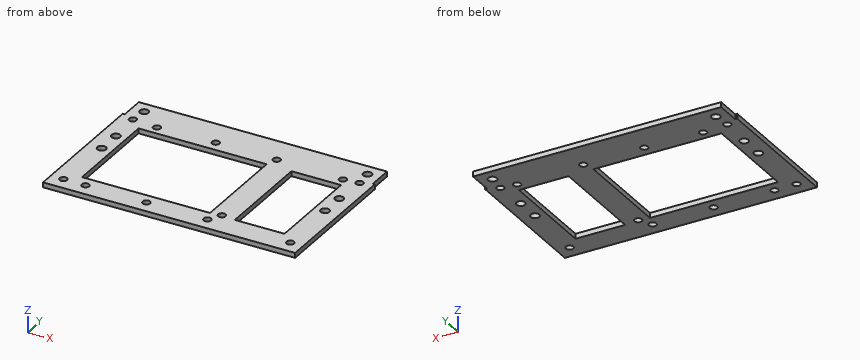
from build123d import *

# Parameters (mm, degrees)
F0_W      = 101.6
F0_H      = 53.34
F1_DEPTH  = 2
F3_D      = 3
F4_W      = 101.6
F4_H      = 3
F4_W_2    = 100
F4_H_2    = 10
F5_DEPTH  = 2
F7_D      = 3.5
F9_D      = 3
F10_W     = 51.6
F10_H     = 40
F10_W_2   = 20
F11_DEPTH = 2.001


with BuildPart() as f1:
    # F0 (on Top) → F1 (new body)
    with BuildSketch(Plane.XY):
        Rectangle(F0_W, F0_H)
    extrude(amount=F1_DEPTH)

    # F3 (through all)
    with Locations(Plane.XY.offset(2)):
        with Locations((-35.56, 24.13), (39.37, 24.13), (45.72, -24.13), (15.24, -19.05), (-36.83, -24.13)):
            Hole(F3_D / 2)

    # F4 (on face) → F5 (join, through all)
    with BuildSketch(Plane.XY.offset(2)):
        with Locations((0, -28.17)):
            Rectangle(F4_W, F4_H)
        with Locations((0, 31.67)):
            Rectangle(F4_W_2, F4_H_2)
    extrude(amount=-F5_DEPTH)

    # F7 (through all)
    with Locations(Plane.XY.offset(2)):
        with Locations((-45, 31.67), (45, 31.67), (-45, 11.67), (-45, 1.67), (45, 11.67), (45, 1.67)):
            Hole(F7_D / 2)

    # F9 (through all)
    with Locations(Plane.XY.offset(2)):
        with Locations((-45.72, -24.13), (-45.72, 24.87), (-12.28, 24.87), (12.28, 24.87), (12.28, -24.13), (-12.28, -24.13), (45.72, 24.87)):
            Hole(F9_D / 2)

    # F10 (on face) → F11 (cut, through all)
    with BuildSketch(Plane(origin=(0, 0, 0), x_dir=(1, 0, 0), z_dir=(0, 0, -1))):
        with Locations((-15, -0.33)):
            Rectangle(F10_W, F10_H)
        with Locations((30.8, -0.33)):
            Rectangle(F10_W_2, F10_H)
    extrude(amount=-F11_DEPTH, mode=Mode.SUBTRACT)


solid = f1.part
Read the model definition and answer for the solid it produces. Units are mm, in the model's axes. Coordinates: 2 decimals unless noted, no trailing zeros. Write each loop counter-clockwise with the first axis right and the second up, starting at its lowest first coordinate (ties: lowest second). Pieces come first, ordered by that corner, then holes. Notation, with made-up numbers: (14.5, 9) - (69.5, 9) arc R18 ccw to (69.5, 13) - close; hole circle Ø10 at (78.5, 18.25). An arc over 180 degrees is marked (long way). One line per question, with ' | ' between items.
Q1. Find section D-D, the plane y = 1.67. Write down the section's boundary in (x, z), plus the area to 3 significant figures.
Result set:
outline: (-50.8, 0) - (-46.75, 0) - (-46.75, 2) - (-50.8, 2) - close; (-43.25, 0) - (-40.8, 0) - (-40.8, 2) - (-43.25, 2) - close; (10.8, 0) - (20.8, 0) - (20.8, 2) - (10.8, 2) - close; (40.8, 0) - (43.25, 0) - (43.25, 2) - (40.8, 2) - close; (46.75, 0) - (50.8, 0) - (50.8, 2) - (46.75, 2) - close | area: 46.0 mm^2
Q2. Each of these flat-tipped pins is pushed along its axis until it touches: P1, Ø6, axis at x = -37, y = -0.5, coming from the -Z side; P2, Ø0.6, axis at x = -50.5, z = 0.5, coming from the +Y side. Where does it stop, or does it pass through?
Result set:
P1: through | P2: y = 26.67
Q3. Consider L1, parallel to X at y = -17, z = 1.75; L2, parallel to X at y = 11.5, z = 1.2; L3, parallel to X at y = -19, z = 0.9. Determine where each line is inside the solid, lowest interval first. Write a range as [from, to].
Result set:
L1: [-50.8, -40.8], [10.8, 20.8], [40.8, 50.8] | L2: [-50.8, -46.74], [-43.26, -40.8], [10.8, 20.8], [40.8, 43.26], [46.74, 50.8] | L3: [-50.8, -40.8], [10.8, 13.74], [16.74, 20.8], [40.8, 50.8]
Q4. Find section A-A, the plane x = -29.5. Write down the section's boundary in (y, z).
Result set:
outline: (-29.67, 0) - (-19.67, 0) - (-19.67, 2) - (-29.67, 2) - close; (20.33, 0) - (36.67, 0) - (36.67, 2) - (20.33, 2) - close
Q5. Find section B-B, the plane y = 31.67. Write down the section's boundary in (x, z), plus the area to 3 significant figures.
Result set:
outline: (-50, 0) - (-46.75, 0) - (-46.75, 2) - (-50, 2) - close; (-43.25, 0) - (43.25, 0) - (43.25, 2) - (-43.25, 2) - close; (46.75, 0) - (50, 0) - (50, 2) - (46.75, 2) - close | area: 186 mm^2
Q6. Find section C-C, the plane z = 1. State how many separate pieces and enclosed holes the cut face has, plus the area to 3 significant figures.
Result set:
separate pieces: 1 | enclosed holes: 20 | area: 3,720 mm^2
